Read the model definition and answer for the solid it produces. Units are mm, in the model's axes. Face numbers are marked on the shaded views. A direction names the side the tool comes from. Give positions to 0.01 mm unless a question says otherwise; leave off trailing zeros. Loops run counter-clockwise (first coordinate to the right, second up) from the corner with the lowest first, then second, coordinate; pieces in that order, holes last. Notation, with made-up numbers: (54, 20.25) -> (67, 20.25) arc R16 ccw to (67, 43.25) -> close; hole circle Ø3 at (28.5, 34). An arc over 180 degrees is marked (long way). Return JSON: item names as keys, results as strings. Group by question number.
Autodesk Fusion 360 part; units mm, degrees
sketch "Sketch1" plane through (0, 0, 0) normal (0, 1, 0) x (1, 0, 0)
  line L0 (0, 0) -> (18.4, 0)
  line L1 (18.4, 0) -> (18.4, -34)
  line L2 (18.4, -34) -> (0, -34)
  line L3 (0, -34) -> (0, 0)
  circle A0 centre (9.2, -24.8) radius 9.2
  circle A1 centre (9.2, -24.8) radius 4.3
  dimension "d1" = 18.4
  dimension "d2" = 34
  dimension "d3" = 4.9
extrude "Extrude2" add sketch "Sketch1" along normal blind 18 contours L0 L1 L3 A0 | A0
fillet "Fillet1" radius 0.5 6 edges at (18.4, 0, 12.4) (9.2, 0, 34) (0, 0, 12.4) (0, 18, 12.4) (9.2, 18, 34) (18.4, 18, 12.4)
sketch "Sketch2" plane through (0, 0, 0) normal (0, 0, 1) x (1, 0, 0)
  line L0 (18.4, 0.5) -> (18.4, 17.5)
sketch "Sketch3" plane through (0, 0, 0) normal (0, 0, 1) x (1, 0, 0)
  circle A0 centre (9.2, 9.2591) radius 2.3
  dimension "d9" = 4.6
extrude "Extrude3" cut sketch "Sketch3" along normal blind 17
extrude "Extrude4" add sketch "Sketch1" along normal blind 7 contours A1
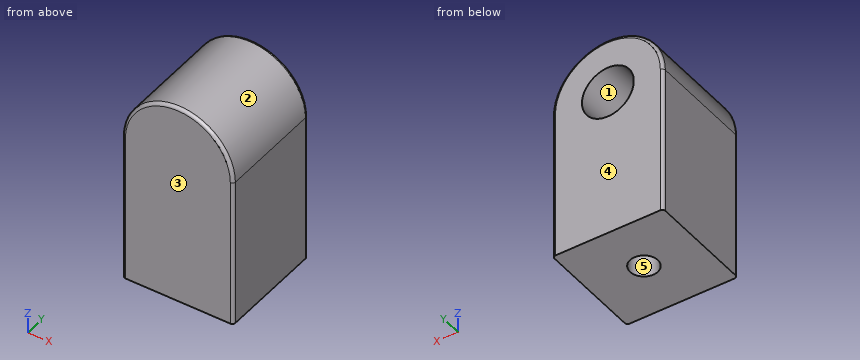
1. Determine the mould class of the marked faces 1, 2 and 3 for opening direction Z: pulls with the +Z half, pulls with the -Z half, needs draft (parallel to the pull), parting line crosses it, or undercut.
2. Section C-C on z = 22.5 is taken. Determine the outline of the cut face in (x, y), then the cut area to 3 significant figures.
3. Flat-ended cylindrical pins translate along their axes: pin 1 Ø10 at (x, z) = (16, 29) entering from -Y; pin 2 Ø7 at (x, z) = (9.2, 24.8) entering from +Y; pin 3 Ø3 at (y, z) = (14, 30.5) entering from -X; pin 4 Ø1.4 at (x, y) = (10, 9) entering from -Z. Find the tip coordinate at first contact, or state that the pin passes through.
4. Section D-D on y = 4 is taken. Determine the outline of the cut face in (x, z).
5. Straight lines are drawn through the part: line 1 (X direction, y = 9.75, z = 24.8); line 2 (Z direction, x = 9.2, y = 12.75); line 3 (Y direction, x = 9.2, z = 4.5). For each, find the intervals that lie inside material, in ascending order. Write a range as from..to.
6. Section A-A on y = 8.5 is taken. Determine the outline of the cut face in (x, z).
7. Section B-B on z = 10.5 is taken. Determine the outline of the cut face in (x, y), then the cut area to 3 significant figures.
8. Which of the six approach directions +Z, -Z, +X, -X, +Y, -Y give full straight-line access (tool end or side, diameter ignored) to the marked faces 4 and 5?
Completed:
{
 "1": {"face 1": "undercut", "face 2": "pulls with the +Z half", "face 3": "needs draft"},
 "2": {"outline": "(0, 0.5) arc R0.5 ccw to (0.5, 0) -> (17.9, 0) arc R0.5 ccw to (18.4, 0.5) -> (18.4, 17.5) arc R0.5 ccw to (17.9, 18) -> (12.83, 18) -> (12.83, 7) -> (5.57, 7) -> (5.57, 18) -> (0.5, 18) arc R0.5 ccw to (0, 17.5) -> close", "area": "251 mm²"},
 "3": {"pin 1": "stops at y = 0", "pin 2": "stops at y = 7", "pin 3": "stops at x = 1.01", "pin 4": "stops at z = 17"},
 "4": {"outline": "(0, 0) -> (18.4, 0) -> (18.4, 24.8) arc R9.2 ccw to (0, 24.8) -> close"},
 "5": {"line 1": "x = 0..4.9, 13.5..18.4", "line 2": "z = 0..20.5, 29.1..34", "line 3": "y = 0..6.96, 11.56..18"},
 "6": {"outline": "(0, 0) -> (7.03, 0) -> (7.03, 17) -> (11.37, 17) -> (11.37, 0) -> (18.4, 0) -> (18.4, 24.8) arc R9.2 ccw to (0, 24.8) -> close; hole circle Ø8.6 at (9.2, 24.8)"},
 "7": {"outline": "(0, 0.5) arc R0.5 ccw to (0.5, 0) -> (17.9, 0) arc R0.5 ccw to (18.4, 0.5) -> (18.4, 17.5) arc R0.5 ccw to (17.9, 18) -> (0.5, 18) arc R0.5 ccw to (0, 17.5) -> close; hole circle Ø4.6 at (9.2, 9.26)", "area": "314 mm²"},
 "8": {"face 4": "+Z, -Z, +X, -X, +Y", "face 5": "-Z"}
}
